Input: part model. Units: mm. Frame: model coordinates. A direction names the side the tool comes from. Round coordinates to 2 decimals unless told otherwise and drop trailing zeros. Order: outer loops, then holes, each group sorted by start corner. A loop starts at its lowest first (then second) coordinate and runs counter-clockwise, first axis right, second up. Notation, with made-up numbers: (49.25, 7) -> (85.25, 7) arc R17 ccw to (85.25, 34) -> close; hole circle Ø7 at (59, -21). An arc over 180 degrees is marked (long way). Use a Markdown table: item, result.
from build123d import *

# Parameters (mm, degrees)
SKETCH1_R                = 4
BOSS_EXTRUDE1_DEPTH      = 6
BOSS_EXTRUDE1_DEPTH_BACK = 6
SKETCH2_W                = 1.5
SKETCH2_H                = 4.5
CUT_EXTRUDE1_DEPTH       = 16


with BuildPart() as part:
    # Sketch1 → Boss-Extrude1 (new body, two sides)
    with BuildSketch(Plane(origin=(0, 0, 0), x_dir=(1, 0, 0), z_dir=(0, 1, 0))) as boss_extrude1_sk:
        with BuildLine():
            Line((-4, 3), (-7.5, 3))
            Line((-7.5, 3), (-7.5, -3))
            Line((-7.5, -3), (-4, -3))
            ThreePointArc((-4, -3), (-3.632728032, -3.435591222), (-3.218284596, -3.826570823))
            Line((-3.218284596, -3.826570823), (6.5, -12))
            Line((6.5, -12), (8.5, -12))
            Line((8.5, -12), (8.5, -1.905552368))
            Line((8.5, -1.905552368), (8.5, 12))
            Line((8.5, 12), (6.5, 12))
            Line((6.5, 12), (-3.218284596, 3.826570823))
            ThreePointArc((-3.218284596, 3.826570823), (-3.632728032, 3.435591222), (-4, 3))
        make_face()
        Circle(SKETCH1_R, mode=Mode.SUBTRACT)
        with BuildLine():
            Line((4.898979486, 1), (6.5, 1))
            Line((6.5, 1), (6.5, 10.040020596))
            Line((6.5, 10.040020596), (0.479918949, 4.976914486))
            ThreePointArc((0.479918949, 4.976914486), (3.34471214, 3.716571095), (4.898979486, 1))
        make_face(mode=Mode.SUBTRACT)
        with BuildLine():
            Line((4.898979486, -1), (6.5, -1))
            Line((6.5, -1), (6.5, -10.040020596))
            Line((6.5, -10.040020596), (0.479918949, -4.976914486))
            ThreePointArc((0.479918949, -4.976914486), (3.34471214, -3.716571095), (4.898979486, -1))
        make_face(mode=Mode.SUBTRACT)
    extrude(amount=BOSS_EXTRUDE1_DEPTH)
    extrude(boss_extrude1_sk.sketch, amount=-BOSS_EXTRUDE1_DEPTH_BACK)

    # Sketch2 → Cut-Extrude1 (cut, through all)
    with BuildSketch(Plane(origin=(0, 0, -3), x_dir=(-1, 0, 0), z_dir=(0, 0, -1))):
        with Locations((5.15, 0)):
            Rectangle(SKETCH2_W, SKETCH2_H)
    extrude(amount=-CUT_EXTRUDE1_DEPTH, mode=Mode.SUBTRACT)


solid = part.part
1) Cut plane D-D on y = 3.5. Return loops of the section in (x, z), and give its area (3 significant figures).
Answer key:
| item | result |
|---|---|
| outline | (-7.5, -3) -> (-4, -3) arc R5 ccw to (-3.22, -3.83) -> (6.5, -12) -> (8.5, -12) -> (8.5, 12) -> (6.5, 12) -> (-3.22, 3.83) arc R5 ccw to (-4, 3) -> (-7.5, 3) -> close; hole circle Ø8 at (0, 0); hole (0.48, -4.98) -> (6.5, -10.04) -> (6.5, -1) -> (4.9, -1) arc R5 cw to start; hole (0.48, 4.98) arc R5 cw to (4.9, 1) -> (6.5, 1) -> (6.5, 10.04) -> close |
| area | 125 mm^2 |
2) Contact query for flat-ended pins moving along their axis: P1, Ø4, axis at x = -6.5, y = -1.5, coming from the +Z side; P2, Ø4, axis at x = -6.5, y = 1, coming from the -Z side; P3, Ø5, axis at y = 4.5, z = -8, coming from the -X side; P4, Ø6.5, axis at x = 0, z = 0, coming from the -Y side. Output: stop coordinate, or through.
Answer key:
| item | result |
|---|---|
| P1 | stops at z = 3 |
| P2 | stops at z = -3 |
| P3 | stops at x = -1.23 |
| P4 | passes through |
3) Draft query along X for faces 5 (the face through (8, 0, -12)), 6 (the face through (8.5, 0, 0)), 7 (the face through (-5, 2.25, 0)), 8 (the face through (1.71, 0.08, -7.97)). Return one class per face: released by +X, released by -X, zero draft, split by the parting line, or undercut.
Answer key:
| item | result |
|---|---|
| face 5 | zero draft |
| face 6 | released by +X |
| face 7 | undercut |
| face 8 | released by -X |
4) Cut plane C-C on x = 1.5. Return loops of the section in (y, z), and give its area (3 significant figures).
Answer key:
| item | result |
|---|---|
| outline | (-6, -7.79) -> (6, -7.79) -> (6, -5.83) -> (-6, -5.83) -> close; (-6, -4.77) -> (6, -4.77) -> (6, -3.71) -> (-6, -3.71) -> close; (-6, 3.71) -> (6, 3.71) -> (6, 4.77) -> (-6, 4.77) -> close; (-6, 5.83) -> (6, 5.83) -> (6, 7.79) -> (-6, 7.79) -> close |
| area | 72.5 mm^2 |
5) Set-up query: faces 1 (the face through (-3.64, 0.08, 3.43)), 2 (the face through (3.53, 0.08, 7.54)), 3 (the face through (-5.9, 0, 0)), 4 (the face through (-6.1, 0.1, -3)). Return all of +Z, -Z, +X, -X, +Y, -Y with unobstructed straight access to the full face (end or side cutting, diameter ignored); none if empty.
Answer key:
| item | result |
|---|---|
| face 1 | +Z, -X, +Y, -Y |
| face 2 | +Y, -Y |
| face 3 | +Z, -Z |
| face 4 | -Z, -X, +Y, -Y |
6) Cut plane A-A on z = 0. Return loops of the section in (x, y).
Answer key:
| item | result |
|---|---|
| outline | (-7.5, -6) -> (-4, -6) -> (-4, 6) -> (-7.5, 6) -> close; (4, -6) -> (8.5, -6) -> (8.5, 6) -> (4, 6) -> close; hole (-5.9, -2.25) -> (-4.4, -2.25) -> (-4.4, 2.25) -> (-5.9, 2.25) -> close |
7) Cut plane B-B on y = -1.75. Return loops of the section in (x, z).
Answer key:
| item | result |
|---|---|
| outline | (-7.5, -3) -> (-5.9, -3) -> (-5.9, 3) -> (-7.5, 3) -> close; (-4.4, -3) -> (-4, -3) arc R5 ccw to (-3.22, -3.83) -> (6.5, -12) -> (8.5, -12) -> (8.5, 12) -> (6.5, 12) -> (-3.22, 3.83) arc R5 ccw to (-4, 3) -> (-4.4, 3) -> close; hole circle Ø8 at (0, 0); hole (0.48, -4.98) -> (6.5, -10.04) -> (6.5, -1) -> (4.9, -1) arc R5 cw to start; hole (0.48, 4.98) arc R5 cw to (4.9, 1) -> (6.5, 1) -> (6.5, 10.04) -> close |
8) Ray query, probe 1 along X at (y, z) = (3.4, 0); probe 2 along Z at (x, y) = (1, -3.25); probe 3 along Z at (x, y) = (5.25, 3). Return the intervals inside material, ascending.
Answer key:
| item | result |
|---|---|
| probe 1 | x = -7.5 to -4, 4 to 8.5 |
| probe 2 | z = -7.37 to -5.41, -4.9 to -3.87, 3.87 to 4.9, 5.41 to 7.37 |
| probe 3 | z = -10.95 to -8.99, -1 to 1, 8.99 to 10.95 |
